Source: CAD feature listing. Evaluate the final solid. Frame: model axes, mm. A direction names the side the tool comes from. Round coordinates to 2 decimals unless told otherwise and drop trailing zeros. Write each loop counter-clockwise with the first axis right and the second up, starting at its lowest first coordinate (ties: lowest second). Pieces come first, ordered by that corner, then holes. Notation, with made-up numbers: M 21.25,62 L 38.25,62 A8 cw 38.25,68 Z; hole C -35.5,-10 d11. An arc over 180 degrees is marked long. Answer in a Markdown table with one row per item.
from build123d import *

# Parameters (mm, degrees)
SKETCH1_R                                           = 25
SKETCH1_R_2                                         = 19
BOSS_EXTRUDE1_DEPTH                                 = 5
SKETCH2_R                                           = 25
BOSS_EXTRUDE2_DEPTH                                 = 10
FILLET1_R                                           = 5
CBORE_FOR_3_BINDING_HEAD_MACHINE_SCREW1_D           = 3.048
CBORE_FOR_3_BINDING_HEAD_MACHINE_SCREW1_CBORE_D     = 5.95376
CBORE_FOR_3_BINDING_HEAD_MACHINE_SCREW1_CBORE_DEPTH = 1.4986
CUT_EXTRUDE1_START                                  = -3
CUT_EXTRUDE1_DEPTH                                  = 10


with BuildPart() as part:
    # Sketch1 → Boss-Extrude1 (new body)
    with BuildSketch(Plane.XY):
        Circle(SKETCH1_R)
        Circle(SKETCH1_R_2, mode=Mode.SUBTRACT)
    extrude(amount=BOSS_EXTRUDE1_DEPTH)

    # Sketch2 → Boss-Extrude2 (add)
    with BuildSketch(Plane.XY.offset(5)):
        Circle(SKETCH2_R)
    extrude(amount=BOSS_EXTRUDE2_DEPTH)

    # Fillet1
    fillet1_edges = [part.edges().sort_by_distance(p)[0] for p in [
        (-25, 0, 15),
        (-19, 0, 5),
    ]]
    fillet(fillet1_edges, radius=FILLET1_R - 0.0001)  # a hair under: the kernel refuses the full size

    # CBORE for #3 Binding Head Machine Screw1 (through all)
    with Locations(Plane.XY.offset(15)):
        with Locations((0, 22.435050854), (0, -22.295918756), (22.400267829, 0), (-22.608965977, 0)):
            CounterBoreHole(CBORE_FOR_3_BINDING_HEAD_MACHINE_SCREW1_D / 2, CBORE_FOR_3_BINDING_HEAD_MACHINE_SCREW1_CBORE_D / 2, CBORE_FOR_3_BINDING_HEAD_MACHINE_SCREW1_CBORE_DEPTH)

    # Sketch15 → Cut-Extrude1 (cut)
    with BuildSketch(Plane(origin=(0, 0, 5), x_dir=(-1, 0, 0), z_dir=(0, 0, -1)).offset(CUT_EXTRUDE1_START)):
        with BuildLine():
            Line((1.676226843, 1.500920907), (2.037127027, 4.807341739))
            Line((2.037127027, 4.807341739), (-0.948609283, 5.133238785))
            Line((-0.948609283, 5.133238785), (-1.309172026, 1.829909453))
            ThreePointArc((-1.309172026, 1.829909453), (-1.94216249, 1.136003901), (-2.236715327, 0.244140421))
            ThreePointArc((-2.236715327, 0.244140421), (-2.141502308, -0.690266516), (-1.673115077, -1.504388892))
            Line((-1.673115077, -1.504388892), (-2.03367782, -4.807718225))
            Line((-2.03367782, -4.807718225), (0.952058491, -5.133615271))
            Line((0.952058491, -5.133615271), (1.312958675, -1.827194439))
            ThreePointArc((1.312958675, -1.827194439), (1.943337692, -1.133992334), (2.236715327, -0.244140421))
            ThreePointArc((2.236715327, -0.244140421), (2.142215878, 0.688048787), (1.676226843, 1.500920907))
        make_face()
    extrude(amount=-CUT_EXTRUDE1_DEPTH, mode=Mode.SUBTRACT)


solid = part.part
Q1. Section D-D (z = 1.5). Return loops of the section in (x, y).
Solutions:
| item | result |
|---|---|
| outline | C 0,0 d50; hole C -22.61,0 d3.05; hole C 0,0 d37.54; hole C 0,-22.3 d3.05; hole C 0,22.44 d3.05; hole C 22.4,0 d3.05 |
Q2. Section A-A (x = 0). State how many separate pieces and enclosed holes the cut face has, and give its area (3 significant figures).
Solutions:
| item | result |
|---|---|
| separate pieces | 3 |
| enclosed holes | 0 |
| area | 398 mm2 |
Q3. Access query for faces 3 (the flat face through (0, 0, 5)), 4 (the flat face through (0, 0, 8)), 5 (the flat face through (-9, -17, 0)). Directions: +Z, -Z, +X, -X, +Y, -Y. A direction counts if a zero-diameter tool reaches every point of the face in a straight line with its end or side. Return the directions, or none.
Solutions:
| item | result |
|---|---|
| face 3 | -Z |
| face 4 | +Z |
| face 5 | -Z, +X, -X, +Y, -Y |
Q4. Material intervals for probe 1 along Z at (x, y) = (12.5, -14); probe 2 along Y at (x, z) = (0, 9.25); probe 3 along Z at (x, y) = (-4.5, 6.5), sorted ascending.
Solutions:
| item | result |
|---|---|
| probe 1 | z = 1.5 to 15 |
| probe 2 | y = -25 to -23.82, -20.77 to -5.03, 5.03 to 20.91, 23.96 to 25 |
| probe 3 | z = 5 to 15 |
Q5. Section C-C (z = 6). Return loops of the section in (x, y), and give its area (3 significant figures).
Solutions:
| item | result |
|---|---|
| outline | C 0,0 d50; hole C -22.61,0 d3.05; hole C 0,-22.3 d3.05; hole C 0,22.44 d3.05; hole C 22.4,0 d3.05 |
| area | 1,930 mm2 |
Q6. Section B-B (z = 9). Return loops of the section in (x, y), and give its area (3 significant figures).
Solutions:
| item | result |
|---|---|
| outline | C 0,0 d50; hole C -22.61,0 d3.05; hole M -2.04,4.81 L -1.68,1.5 A2.25 ccw -1.31,-1.83 L -0.95,-5.13 L 2.03,-4.81 L 1.67,-1.5 A2.25 ccw 1.31,1.83 L 0.95,5.13 Z; hole C 0,-22.3 d3.05; hole C 0,22.44 d3.05; hole C 22.4,0 d3.05 |
| area | 1,900 mm2 |
Q7. Pull-direction query (Y, two-part tool) for faces 1 (the flat face through (-0.565, 4.968, 11.451)), 2 (the flat face through (4, 0, 15)); classes: pulls with the +Y half, pulls with the -Y half, needs draft (parallel to the pull), parting line crosses it, or undercut.
Solutions:
| item | result |
|---|---|
| face 1 | undercut |
| face 2 | needs draft |
Q8. Contact query for flat-ended pins moving along their axis: pin 1 Ø1 at (x, z) = (2, 8) entering from +Y; pin 2 Ø2 at (x, y) = (0, -2) entering from +Z; pin 3 Ø3 at (x, z) = (-5.5, 3.5) entering from -Y; pin 4 Ø2.5 at (x, y) = (0, -22.3) entering from -Z. Output: stop coordinate, or through.
Solutions:
| item | result |
|---|---|
| pin 1 | stops at y = 24.95 |
| pin 2 | stops at z = 8 |
| pin 3 | stops at y = -24.68 |
| pin 4 | passes through |
